```python
from build123d import *

# Parameters (mm, degrees)
SKETCH1_W               = 44.85
SKETCH1_H               = 44.85
SKETCH1_W_2             = 38.5
SKETCH1_H_2             = 38.5
BOSS_EXTRUDE1_DEPTH     = 19.25
SKETCH2_W               = 44.85
SKETCH2_H               = 44.85
BOSS_EXTRUDE2_DEPTH     = 3.175
SKETCH3_W               = 44.85
SKETCH3_H               = 44.85
BOSS_EXTRUDE3_DEPTH     = 3.175
SKETCH5_R               = 12.7
CUT_EXTRUDE1_DEPTH      = 3.175
CUT_EXTRUDE2_START      = 22.425
SKETCH6_R               = 10
CUT_EXTRUDE2_DEPTH      = 41.675
SKETCH8_W               = 44.85
SKETCH8_H               = 44.85
SKETCH8_R               = 2.2225
BOSS_EXTRUDE4_DEPTH     = 6.35
SKETCH9_R               = 3.4925
CUT_EXTRUDE4_DEPTH      = 6.35
CUT_EXTRUDE5_REACH      = 62.226
SKETCH10_W              = 38.5
SKETCH10_H              = 38.5
BOSS_EXTRUDE5_DEPTH     = 12.7
BOSS_EXTRUDE6_DEPTH     = 5.75
BOSS_EXTRUDE7_DEPTH     = 5.75
SKETCH15_W              = 56.35
SKETCH15_H              = 44.85
SKETCH15_W_2            = 38.5
SKETCH15_H_2            = 38.5
BOSS_EXTRUDE8_DEPTH     = 2.575
CUT_EXTRUDE3_DEPTH      = 54.437785087
CUT_EXTRUDE3_DEPTH_BACK = 54.437785087
SKETCH7_R               = 12.7


with BuildPart() as part:
    # Sketch1 → Boss-Extrude1 (new, symmetric)
    with BuildSketch(Plane(origin=(0, 0, 0), x_dir=(1, 0, 0), z_dir=(0, 1, 0))):
        Rectangle(SKETCH1_W, SKETCH1_H)
        Rectangle(SKETCH1_W_2, SKETCH1_H_2, mode=Mode.SUBTRACT)
    extrude(amount=BOSS_EXTRUDE1_DEPTH, both=True)

    # Sketch2 → Boss-Extrude2 (add)
    with BuildSketch(Plane(origin=(0, 19.25, 0), x_dir=(1, 0, 0), z_dir=(0, 1, 0))):
        Rectangle(SKETCH2_W, SKETCH2_H)
    extrude(amount=BOSS_EXTRUDE2_DEPTH)

    # Sketch3 → Boss-Extrude3 (add)
    with BuildSketch(Plane.XZ.offset(19.25)):
        Rectangle(SKETCH3_W, SKETCH3_H)
    extrude(amount=BOSS_EXTRUDE3_DEPTH)

    # Sketch5 → Cut-Extrude1 (cut)
    with BuildSketch(Plane(origin=(0, -22.425, -22.425), x_dir=(1, 0, 0), z_dir=(0, 1, 0))):
        with Locations(Location((0, -22.425, 0), (0, 0, 90))):
            Circle(SKETCH5_R)
    extrude(amount=CUT_EXTRUDE1_DEPTH, mode=Mode.SUBTRACT)

    # Sketch6 → Cut-Extrude2 (cut)
    with BuildSketch(Plane(origin=(0, 0, 0), x_dir=(1, 0, 0), z_dir=(0, 1, 0)).offset(CUT_EXTRUDE2_START)):
        with Locations(Location((0, 0, 0), (0, 0, 270))):
            Circle(SKETCH6_R)
    extrude(amount=-CUT_EXTRUDE2_DEPTH, mode=Mode.SUBTRACT)

    # Sketch8 → Boss-Extrude4 (add)
    with BuildSketch(Plane(origin=(0, 0, -22.425), x_dir=(-1, 0, 0), z_dir=(0, 0, -1))):
        Rectangle(SKETCH8_W, SKETCH8_H)
        with Locations((-12.7, 12.7)):
            Circle(SKETCH8_R, mode=Mode.SUBTRACT)
        with Locations((0, 12.7)):
            Circle(SKETCH8_R, mode=Mode.SUBTRACT)
        with Locations((12.7, 12.7)):
            Circle(SKETCH8_R, mode=Mode.SUBTRACT)
        Circle(SKETCH8_R, mode=Mode.SUBTRACT)
        with Locations((12.7, 0)):
            Circle(SKETCH8_R, mode=Mode.SUBTRACT)
        with Locations((0, -12.7)):
            Circle(SKETCH8_R, mode=Mode.SUBTRACT)
        with Locations((12.7, -12.7)):
            Circle(SKETCH8_R, mode=Mode.SUBTRACT)
        with Locations((-12.7, 0)):
            Circle(SKETCH8_R, mode=Mode.SUBTRACT)
        with Locations((-12.7, -12.7)):
            Circle(SKETCH8_R, mode=Mode.SUBTRACT)
    extrude(amount=BOSS_EXTRUDE4_DEPTH)

    # Sketch9 → Cut-Extrude4 (cut)
    with BuildSketch(Plane.XY.offset(-19.25)):
        with Locations((12.7, 12.7)):
            Circle(SKETCH9_R)
        with Locations((0, 12.7)):
            Circle(SKETCH9_R)
        with Locations((-12.7, 12.7)):
            Circle(SKETCH9_R)
        Circle(SKETCH9_R)
        with Locations((-12.7, 0)):
            Circle(SKETCH9_R)
        with Locations((0, -12.7)):
            Circle(SKETCH9_R)
        with Locations((-12.7, -12.7)):
            Circle(SKETCH9_R)
        with Locations((12.7, 0)):
            Circle(SKETCH9_R)
        with Locations((12.7, -12.7)):
            Circle(SKETCH9_R)
    extrude(amount=-CUT_EXTRUDE4_DEPTH, mode=Mode.SUBTRACT)

    # Sketch10 → Cut-Extrude5 (cut, up to next)
    with BuildSketch(Plane.XY.offset(22.425), mode=Mode.PRIVATE) as cut_extrude5_sk1:
        Rectangle(SKETCH10_W, SKETCH10_H)
    cut_extrude5_tool1 = extrude(cut_extrude5_sk1.sketch, amount=-CUT_EXTRUDE5_REACH, mode=Mode.PRIVATE) & part.part
    add(cut_extrude5_tool1.solids().sort_by_distance((0, 0, 22.425))[0], mode=Mode.SUBTRACT)

    # Sketch11 → Boss-Extrude5 (add)
    with BuildSketch(Plane(origin=(0, 22.425, 0), x_dir=(1, 0, 0), z_dir=(0, 1, 0))):
        with BuildLine():
            Line((-28.175, 0), (-25, 0))
            ThreePointArc((-25, 0), (0, 25), (25, 0))
            Line((25, 0), (28.175, 0))
            Line((28.175, 0), (28.175, 28.775))
            Line((28.175, 28.775), (-28.175, 28.775))
            Line((-28.175, 28.775), (-28.175, 0))
        make_face()
    extrude(amount=BOSS_EXTRUDE5_DEPTH)

    # Sketch12 → Boss-Extrude6 (add)
    with BuildSketch(Plane.ZY.offset(22.425)):
        Polygon((-11.050763548, 22.425), (-28.775, 22.425), (-28.775, -22.425), (22.425, -22.425), (22.425, 22.425), align=None)
    extrude(amount=BOSS_EXTRUDE6_DEPTH)

    # Sketch13 → Boss-Extrude7 (add)
    with BuildSketch(Plane(origin=(22.425, 0, 0), x_dir=(0, 0, -1), z_dir=(1, 0, 0))):
        Polygon((-22.425, 22.425), (-22.425, -22.425), (28.775, -22.425), (28.775, 22.425), (11.050763548, 22.425), align=None)
    extrude(amount=BOSS_EXTRUDE7_DEPTH)

    # Sketch15 → Boss-Extrude8 (add)
    with BuildSketch(Plane.XY.offset(22.425)):
        Rectangle(SKETCH15_W, SKETCH15_H)
        Rectangle(SKETCH15_W_2, SKETCH15_H_2, mode=Mode.SUBTRACT)
    extrude(amount=BOSS_EXTRUDE8_DEPTH)

    # Sketch7 → Cut-Extrude3 (cut, two sides: drawn at the far end of the back side and taken through both)
    with BuildSketch(Plane.ZY.offset(-CUT_EXTRUDE3_DEPTH_BACK)):
        Circle(SKETCH7_R)
    extrude(amount=CUT_EXTRUDE3_DEPTH + CUT_EXTRUDE3_DEPTH_BACK, mode=Mode.SUBTRACT)


solid = part.part
```
CAD build for the part. Positions are in the model's coordinates, mm. A direction names the side the tool comes from. Round coordinates to 2 decimals unless told otherwise and drop trailing zeros. Order: outer loops, then holes, each group sorted by start corner. A loop starts at its lowest first (then second) coordinate and runs counter-clockwise, first axis right, second up. Notation, with made-up numbers: (31, 46) - (54, 46) arc R25 ccw to (54, 67) - close; hole circle Ø2 at (65, 79). An arc over 180 degrees is marked (long way). Answer as CSV lines item,"result". Start each with the question number.
1. Tool access for faces 4 (the face through (15, -13.4, -25.6)), 5 (the face through (-23.65, -12.4, -2.75)): list every direction of +Z, -Z, +X, -X, +Y, -Y with a clear straight run to the whole face (end or side of a thin tool).
2. Pin check, flat tips, straight feed: pin 1 (2 mm diameter, centred on x = 4.5, z = 7, fed in from -Y); pin 2 (1 mm diameter, centred on x = -10.5, y = -9.5, fed in from +Z); pin 3 (2.5 mm diameter, centred on x = 27, y = 30, fed in from +Z); pin 4 (2 mm diameter, centred on x = 1, y = 1.5, fed in from +Z). Stop position of each tip, or through.
3. Pull direction X, two halves, no side cores. Call faces 1 (the face through (28.175, 12, -8)), 2 (the face through (-16.19, 0.15, -22.38)), 3 (the face through (-27, 29, 0)): +X half, -X half, draft (parallel to the pull), parting line (faces both ways), or undercut.
4. Saw through at B-B, the plane x = 6. Write the cut outline in (y, z) (3 decimals), and give its area (3 significant figures).
5. Saw through at D-D, the plane x = 22.5. Write the cut outline in (y, z) (3 decimals).
6. Saw through at C-C, the plane z = 17.5. Write the cut outline in (x, y) (3 decimals).
7. Drill centre lines: L1, parallel to Y at x = 12.7, z = -21 (1 decimal); L2, parallel to X at y = -12.7, z = -27.7 (1 decimal); L3, parallel to Y at x = 19, z = 6 (3 decimals). Where is each one in solid material? Low to high. Write a range as [from, to].
8. Saw through at A-A, the plane y = 21. Write the cut outline in (x, z) (3 decimals).
Model answer:
1,face 4,"+Z"
1,face 5,"+X, -X"
2,pin 1,"passes through"
2,pin 2,"stops at z = -19.25"
2,pin 3,"stops at z = 0"
2,pin 4,"stops at z = -25.6"
3,face 1,"+X half"
3,face 2,"undercut"
3,face 3,"draft"
4,outline,"(-22.425, -28.775) - (35.125, -28.775) - (35.125, -24.269) - (22.425, -24.269) - (22.425, -8) - (19.25, -8) - (19.25, -19.25) - (-19.25, -19.25) - (-19.25, -11.193) - (-22.425, -11.193) - close; (-22.425, 11.193) - (-19.25, 11.193) - (-19.25, 25) - (-22.425, 25) - close; (19.25, 8) - (22.425, 8) - (22.425, 25) - (19.25, 25) - close"
4,area,"644 mm²"
5,outline,"(-22.425, -28.775) - (35.125, -28.775) - (35.125, -10.897) - (22.425, -10.897) - (22.425, 25) - (-22.425, 25) - close; hole circle Ø25.4 at (0, 0)"
6,outline,"(-28.175, -22.425) - (28.175, -22.425) - (28.175, 22.425) - (-28.175, 22.425) - close; hole (-19.25, -19.25) - (19.25, -19.25) - (19.25, 19.25) - (-19.25, 19.25) - close"
7,L1,"y = [-22.4, -16.2], [-9.2, -3.5], [3.5, 9.2], [16.2, 22.4]"
7,L2,"x = [-28.2, -14.9], [-10.5, -2.2], [2.2, 10.5], [14.9, 28.2]"
7,L3,"y = [-22.425, -19.25], [19.25, 22.425]"
8,outline,"(-28.175, -28.775) - (28.175, -28.775) - (28.175, 25) - (-28.175, 25) - close; hole circle Ø20 at (0, 0)"
